from build123d import *

# Parameters (mm, degrees)
F0_W     = 1200
F0_H     = 600
F1_DEPTH = 250
F3_DEPTH = 250
F4_W     = 400
F4_H     = 260
F5_DEPTH = 250.001
F6_W     = 400
F6_H     = 260
F7_DEPTH = 250.001


with BuildPart() as f1:
    # F0 (on Top) → F1 (new body)
    with BuildSketch(Plane.XY):
        Rectangle(F0_W, F0_H)
    extrude(amount=F1_DEPTH)

    # F2 (on face) → F3 (join)
    with BuildSketch(Plane.XY.offset(250)):
        Polygon((300, 0), (0, 300), (-300, 0), (0, -300), align=None)
    extrude(amount=F3_DEPTH)

    # F4 (on face) → F5 (cut, through all)
    with BuildSketch(Plane.XY.offset(250)):
        with Locations((-600, 0)):
            Rectangle(F4_W, F4_H)
    extrude(amount=-F5_DEPTH, mode=Mode.SUBTRACT)

    # F6 (on face) → F7 (cut, through all)
    with BuildSketch(Plane.XY.offset(250)):
        with Locations((600, 0)):
            Rectangle(F6_W, F6_H)
    extrude(amount=-F7_DEPTH, mode=Mode.SUBTRACT)


solid = f1.part
Model file for the job. Use its own axes, mm. A direction names the side the tool comes from. Give positions to 0.01 mm unless a question says otherwise; leave off trailing zeros. Order: outer loops, then holes, each group sorted by start corner. A loop starts at its lowest first (then second) coordinate and runs counter-clockwise, first axis right, second up. Notation, with made-up numbers: (64, -31) - (122, -31) arc R22 ccw to (122, -11) - close; hole circle Ø5 at (22, 74.5). An arc over 180 degrees is marked (long way). Return JSON: item names as keys, results as strings.
1) Cut at A-A, the plane x = -461. Give the cut face in (y, z).
Geometry says:
{"outline": "(-300, 0) - (-130, 0) - (-130, 250) - (-300, 250) - close; (130, 0) - (300, 0) - (300, 250) - (130, 250) - close"}
2) Probe line 1 (Y direction, x = -513, z = 225); line 2 (Z direction, x = 355.5, y = 146); line 3 (X direction, y = -15, z = 96). List the from-to ranges inside material, lowest first. Write a range as from..to.
Geometry says:
{"line 1": "-300..-130, 130..300", "line 2": "0..250", "line 3": "-400..400"}
3) Cut at D-D, the plane z = 139. Give the cut face in (x, y).
Geometry says:
{"outline": "(-600, -300) - (600, -300) - (600, -130) - (400, -130) - (400, 130) - (600, 130) - (600, 300) - (-600, 300) - (-600, 130) - (-400, 130) - (-400, -130) - (-600, -130) - close"}
4) Pull direction Y, two halves, no side cores. Call faces 5 (the flat face through (-148, 152, 373)), 6 (the flat face through (-8, -300, 123)), 7 (the flat face through (-8, 4, 0)), 8 (the flat face through (400, -2, 127)): pulls with the +Y half, pulls with the -Y half, needs draft (parallel to the pull), parting line crosses it, or undercut.
Geometry says:
{"face 5": "pulls with the +Y half", "face 6": "pulls with the -Y half", "face 7": "needs draft", "face 8": "undercut"}
5) Cut at B-B, the plane y = -211.5. Give the cut face in (x, z), plus the area to 3 significant figures.
Geometry says:
{"outline": "(-600, 0) - (600, 0) - (600, 250) - (88.5, 250) - (88.5, 500) - (-88.5, 500) - (-88.5, 250) - (-600, 250) - close", "area": "344,000 mm²"}
6) Cut at C-C, the plane x = 279. Give the cut face in (y, z).
Geometry says:
{"outline": "(-300, 0) - (300, 0) - (300, 250) - (21, 250) - (21, 500) - (-21, 500) - (-21, 250) - (-300, 250) - close"}
7) Flat gauge pins, fed straight in: P1, Ø3, axis at y = 166, z = 341.5, coming from the +X side; P2, Ø4, axis at y = 66, z = 412, coming from the -X side; P3, Ø8, axis at y = -182, z = 374.5, coming from the +X side. Where does each tip first touch, or does it go through?
Geometry says:
{"P1": "x = 135.5", "P2": "x = -236", "P3": "x = 122"}
8) 3-axis set-ups, long thin cutter, end or side, ignore diameter. For faces 1 (the flat face through (362, 4, 250)), 2 (the flat face through (152, 148, 373)), 3 (the flat face through (-400, -2, 127)), 4 (the flat face through (499, -130, 127)): which of +Z, -Z, +X, -X, +Y, -Y reach the whole face in a straight line?
Geometry says:
{"face 1": "+Z, +X", "face 2": "+Z, +X, +Y", "face 3": "+Z, -Z, -X", "face 4": "+Z, -Z, +X"}
